from build123d import *

# Parameters (mm, degrees)
SKETCH2_R           = 25
BOSS_EXTRUDE1_DEPTH = 4
SKETCH3_R           = 25
SKETCH3_R_2         = 1
BOSS_EXTRUDE2_DEPTH = 2
CUT_EXTRUDE1_DEPTH  = 36.860842154
CIRPATTERN1_COUNT   = 10


with BuildPart() as part:
    # Sketch2 → Boss-Extrude1 (new body)
    with BuildSketch(Plane.XY):
        Circle(SKETCH2_R)
        with BuildLine():
            Line((1.9, -1.918332609), (1.9, 1.918332609))
            ThreePointArc((1.9, 1.918332609), (0, 2.7), (-1.9, 1.918332609))
            Line((-1.9, 1.918332609), (-1.9, -1.918332609))
            ThreePointArc((-1.9, -1.918332609), (0, -2.7), (1.9, -1.918332609))
        make_face(mode=Mode.SUBTRACT)
    extrude(amount=-BOSS_EXTRUDE1_DEPTH)

    # Sketch3 → Boss-Extrude2 (add)
    with BuildSketch(Plane(origin=(0, 0, -4), x_dir=(-1, 0, 0), z_dir=(0, 0, -1))):
        with Locations(Location((0, 0, 0), (0, 0, 180))):
            Circle(SKETCH3_R)
        Circle(SKETCH3_R_2, mode=Mode.SUBTRACT)
    extrude(amount=BOSS_EXTRUDE2_DEPTH)

    # Sketch4 → Cut-Extrude1 (cut, symmetric)
    with BuildSketch(Plane.XY):
        with BuildLine():
            Line((-0.857142857, 18), (0.857142857, 18))
            Line((0.857142857, 18), (0.998868138, 20.976230892))
            ThreePointArc((0.998868138, 20.976230892), (0, 21), (-0.998868138, 20.976230892))
            Line((-0.998868138, 20.976230892), (-0.857142857, 18))
        make_face()
    cut_extrude1 = extrude(amount=CUT_EXTRUDE1_DEPTH, both=True, mode=Mode.SUBTRACT)

    # CirPattern1: Cut-Extrude1 ×10 about axis
    cirpattern1_axis = Axis((0, 0, 0), (0, 0, 1))
    for i in range(1, CIRPATTERN1_COUNT):
        add(cut_extrude1.rotate(cirpattern1_axis, i * 360 / CIRPATTERN1_COUNT), mode=Mode.SUBTRACT)


solid = part.part
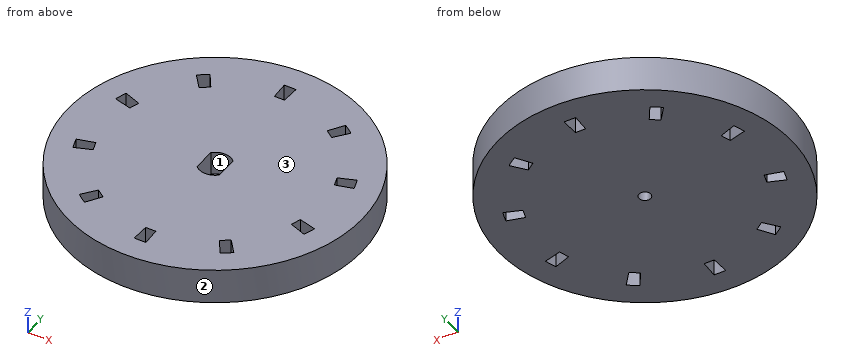
CAD build for the part. Positions are in the model's coordinates, mm. Face numbers are marked on the shaded views. Round coordinates to 2 decimals unless told otherwise and drop trailing zeros. Loops run counter-clockwise (first coordinate to the right, second up) from the corner with the lowest first, then second, coordinate; pieces in that order, holes last.
(1) Wall check: line 1 along Y through (x, z) = (0, -4.8); line 2 along X through (y, z) = (15, -5.25); line 3 along X through (y, z) = (6, -5.25). Give the ranges that are in metal, low to high.
(2) Cut at B-B (y = 0). Give the cut face in (x, z).
(3) Two-plate mould, pull along Y, no slides. Class the marked faces 1, 2 and 3: +Y half, -Y half, draft (parallel to the pull), parting line (faces both ways), or undercut.
(4) Cut at C-C (z = -5). State how many separate pieces and enclosed holes the cut face has, plus the area to 3 significant figures.
(5) Cut at A-A (x = 0). Give the cut face in (y, z).
(6) Drop flat-ended pins along their axis: pin 1 (3 mm diameter, centred on x = 6, z = -3, fed in from -Y); pin 2 (1.9 mm diameter, centred on x = 0.5, z = -3, fed in from +Y); pin 3 (3 mm diameter, centred on x = 1.5, z = -5.5, fed in from -Y). Give the stop position or say it passes through.
(7) Cut at D-D (x = 7). Give the cut face in (y, z), plus the area to 3 significant figures.
Findings below:
1. line 1: y = -25 to -21, -18 to -1, 1 to 18, 21 to 25
1. line 2: x = -20 to -12.03, -9.98 to 9.98, 12.03 to 20
1. line 3: x = -24.27 to -20.12, -16.98 to 16.98, 20.12 to 24.27
2. outline: (-25, -6) - (-1, -6) - (-1, -4) - (-1.9, -4) - (-1.9, 0) - (-25, 0) - close; (1, -6) - (25, -6) - (25, 0) - (1.9, 0) - (1.9, -4) - (1, -4) - close
3. face 1: undercut
3. face 2: parting line
3. face 3: draft
4. separate pieces: 1
4. enclosed holes: 11
4. area: 1,900 mm2
5. outline: (-25, -6) - (-21, -6) - (-21, 0) - (-25, 0) - close; (-18, -6) - (-1, -6) - (-1, -4) - (-2.7, -4) - (-2.7, 0) - (-18, 0) - close; (1, -6) - (18, -6) - (18, 0) - (2.7, 0) - (2.7, -4) - (1, -4) - close; (21, -6) - (25, -6) - (25, 0) - (21, 0) - close
6. pin 1: stops at y = -24.59
6. pin 2: stops at y = 25
6. pin 3: stops at y = -25
7. outline: (-24, -6) - (24, -6) - (24, 0) - (-24, 0) - close
7. area: 288 mm2
